Can you work these out from the model? Positions are in its coordinate system, mm. A direction names the side the tool comes from. Coordinates: 2 decimals unless noted, no trailing zeros. Order: outer loops, then holes, each group sorted by start corner. A loop starts at its lowest first (then second) coordinate and runs counter-clockwise, first axis right, second up. Notation, with made-up numbers: (-28.5, 23.5) -> (28.5, 23.5) arc R22 cw to (28.5, 33.5) -> close; hole circle Ø11 at (-40, 44). An arc over 180 degrees is marked (long way). Use a Markdown table: item, result. Add a question column.
1. Suppose I cut it at A-A, the plane z = 223. List the corners of the cut face in (x, y) for me, then the cut area to 3 significant figures.
2. For faces 4 (the flat face through (1.92, -0.15, 391.4)), 5 (the flat face through (21.977, -25.266, 194.36)), which set-ups out of +Z, -Z, +X, -X, +Y, -Y let a thin tool reach every point of the face, with its end or its side?
3. Suppose I cut it at C-C, the plane y = 9.5. List the corners of the cut face in (x, z) for me, then the cut area to 3 significant figures.
4. If I drill on line 1 along X through (y, z) = (-16.5, 235); line 2 along Y through (x, z) = (8.5, 220); line 3 along Y through (x, z) = (21, 102.5), over which ranges is the centre line in solid material (lowest first)? Write a range as from..to.
5. For pin 1 Ø10 at (x, y) = (13, -17) entering from -Z; pin 2 Ø18.5 at (y, z) = (3.5, 276.5) entering from +X; pin 3 Ø5 at (x, z) = (8.5, 68) entering from +Y, each with a flat end and sliding along its axis, tell me the tip position at first contact or that it passes through.
6. Suppose I cut it at D-D, the plane z = 387. List the corners of the cut face in (x, y) for me.
7. We'd pull the mould along Y, two halves only. Please class faces 1 (the flat face through (21.977, 25.266, 240.089)), 2 (the flat face through (3.25, 19.39, 63.65)), 3 (the flat face through (18, -32.5, 195)): pulls with the +Y half, pulls with the -Y half, needs draft (parallel to the pull), parting line crosses it, or undercut.
8. Suppose I cut it at B-B, the plane z = 55. List the corners of the cut face in (x, y) for me.
Autodesk Inventor part; units mm, degrees
ref_plane "Начальная плоскость" through (0, 0, 23.4485) normal (0, 0, 1) x (1, 0, 0)
ref_plane "Конечная плоскость" through (0, 0, 422.7409) normal (0, 0, 1) x (1, 0, 0)
ref_plane "РабПлоскость8" through (0, -195.6097, 203.8212) normal (0, -0.6924, 0.7215) x (1, 0, 0)
ref_plane "Начальная плоскость" through (0, 0, 23.4485) normal (0, 0, 1) x (1, 0, 0)
ref_plane "Конечная плоскость" through (0, 0, 422.7409) normal (0, 0, 1) x (1, 0, 0)
sketch "Эскиз" plane through (0, 0, 0) normal (0, 0, 1) x (1, 0, 0)
  line L0 (36, -32.5) -> (0, -32.5)
  line L1 (36, -32.5) -> (36, -28.696)
  line L2 (33.6994, -26.2039) -> (9.9215, -24.3017)
  line L3 (4.4, -18.3208) -> (4.4, 18.3208)
  line L4 (33.6994, 26.2039) -> (9.9215, 24.3017)
  line L5 (36, 28.696) -> (36, 32.5)
  line L6 (0, 32.5) -> (36, 32.5)
  line L7 (0, -32.5) -> (0, 32.5)
  arc A0 (4.4, -18.3208) -> (9.9215, -24.3017) centre (10.4, -18.3208) ccw
  arc A1 (9.9215, 24.3017) -> (4.4, 18.3208) centre (10.4, 18.3208) ccw
  arc A2 (36, -28.696) -> (33.6994, -26.2039) centre (33.5, -28.696) ccw
  arc A3 (33.6994, 26.2039) -> (36, 28.696) centre (33.5, 28.696) ccw
  line L8 (0, 45.5) -> (0, -45.5) construction
  line L9 (-7.2974, 0) -> (43.7847, 0) construction
  point P0 (36, -26.388)
  point P1 (4.4, -23.86)
  point P2 (4.4, 23.86)
  point P3 (36, 26.388)
  dimension "d3" = 36
  dimension "d5" = 4.4
  dimension "d7" = 65
  dimension "d9" = 8.64
  dimension "d11" = 8.64
  dimension "d13" = 6.112
  dimension "d15" = 6.112
  dimension "d22" = 6
  dimension "d23" = 2.5
  dimension "d24" = 32.5
  dimension "d25" = 0
extrude "Тело" add sketch "Эскиз" along normal up to surface (399.2924 mm away) from surface at 23.4485
sketch "Sketch3" plane through (0, 0, 0) normal (0, 0, 1) x (1, 0, 0)
  line L0 (0, 0) -> (10, 0)
ref_plane "Work Plane7" through (0, 0, 0) normal (0, -1, 0) x (1, 0, 0)
sketch "Sketch4" plane through (0, 0, 0) normal (0, -1, 0) x (1, 0, 0)
  line L0 (-2, 23.4485) -> (12, 23.4485)
  line L1 (-2, 422.7409) -> (12, 422.7409)
  dimension "d29" = 399.2924
ref_plane "РабПлоскость8" through (0, -195.6097, 203.8212) normal (0, -0.6924, 0.7215) x (1, 0, 0)
split "Разделение1" plane through (0, -195.6097, 203.8212) removes the side toward (0, -0.6924, 0.7215)
ref_plane "РабПлоскость9" through (36, -22.5038, 23.4485) normal (0, 0.6924, -0.7215) x (1, 0, 0)
split "Разделение2" plane through (36, -22.5038, 23.4485) removes the side toward (0, 0.6924, -0.7215)
ref_plane "РабПлоскость10" through (-29, -461.8467, 481.2345) normal (0, -0.7215, -0.6924) x (1, 0, 0)
split "Разделение3" plane through (-29, -461.8467, 481.2345) removes the side toward (0, -0.7215, -0.6924)
equation "\"d3\" = b"
equation "\"d7\" = ParH"
equation "\"d22\" = R"
equation "\"d23\" = R1"
equation "\"d24\" = 0.5 * d7"
equation "\"d16\" = G_L"
equation "\"R1\" = 2.5"
equation "\"R\" = 6"
equation "\"t1\" = 4.4"
equation "\"t2\" = 7.2"
equation "\"ParH\" = 65"
equation "\"b\" = 36"
equation "\"msp_x1\" = 0.04 * b"
equation "\"msp_x2\" = -0.08 * t1 + 0.04 * b"
equation "\"G_L\" = d29"
equation "\"ex\" = 0"
equation "\"G_OFFSET_START\" = -23.44846"
equation "\"G_OFFSET_END\" = -58.90056"
equation "\"d26\" = -G_OFFSET_START"
equation "\"d27\" = G_OFFSET_END + B_L"
equation "\"B_L\" = 481.64146"
properties part number "Швеллер 6.5U-399,29 ГОСТ 8240-97" material "Сталь, мягкая"
Worked out:
| question | item | result |
|---|---|---|
| 1 | outline | (0, -32.5) -> (36, -32.5) -> (36, -28.7) arc R2.5 ccw to (33.7, -26.2) -> (9.92, -24.3) arc R6 cw to (4.4, -18.32) -> (4.4, 18.32) arc R6 cw to (9.92, 24.3) -> (33.7, 26.2) arc R2.5 ccw to (36, 28.7) -> (36, 32.5) -> (0, 32.5) -> close |
| 1 | area | 763 mm² |
| 2 | face 4 | +Z, +X, -X, -Y |
| 2 | face 5 | +Z, -Z, +X |
| 3 | outline | (0, 54.16) -> (4.4, 54.16) -> (4.4, 400.66) -> (0, 400.66) -> close |
| 3 | area | 1,520 mm² |
| 4 | line 1 | x = 0..4.4 |
| 4 | line 2 | y = -32.5..-24.01, 24.01..32.5 |
| 4 | line 3 | y = -32.5..-25.19, 25.19..32.5 |
| 5 | pin 1 | passes through |
| 5 | pin 2 | stops at x = 4.4 |
| 5 | pin 3 | stops at y = 26.53 |
| 6 | outline | (0, -4.73) -> (4.4, -4.73) -> (4.4, 18.32) arc R6 cw to (9.92, 24.3) -> (33.7, 26.2) arc R2.5 ccw to (36, 28.7) -> (36, 32.5) -> (0, 32.5) -> close |
| 7 | face 1 | undercut |
| 7 | face 2 | pulls with the +Y half |
| 7 | face 3 | pulls with the -Y half |
| 8 | outline | (0, -32.5) -> (36, -32.5) -> (36, -28.7) arc R2.5 ccw to (33.7, -26.2) -> (9.92, -24.3) arc R6 cw to (4.4, -18.32) -> (4.4, 10.37) -> (0, 10.37) -> close |
